Input: part model. Units: mm. Frame: model coordinates. Face numbers are marked on the shaded views. A direction names the side the tool comes from. Give positions to 0.01 mm unless a question says otherwise; leave off trailing zeros. Loops run counter-clockwise (first coordinate to the right, second up) from the corner with the lowest first, then second, coordinate; pieces in that order, holes last.
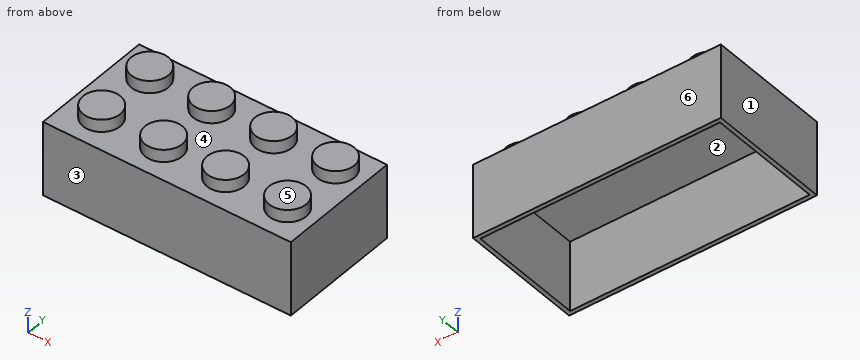
from build123d import *

# Parameters (mm, degrees)
F0_W     = 60
F0_H     = 30
F1_DEPTH = 18
F2_T     = -1
F3_R     = 4.5
F4_DEPTH = 3


with BuildPart() as f1:
    # F0 (on Top) → F1 (new body)
    with BuildSketch(Plane.XY):
        with Locations((30, 15)):
            Rectangle(F0_W, F0_H)
    extrude(amount=F1_DEPTH)

    # F2
    f2_openings = [f1.faces().sort_by_distance(p)[0] for p in [
        (30, 15, 0),
    ]]
    offset(amount=F2_T, openings=f2_openings)

    # F3 (on face) → F4 (join)
    with BuildSketch(Plane.XY.offset(18)):
        with Locations((8, 8)):
            Circle(F3_R)
        with Locations((23, 8)):
            Circle(F3_R)
        with Locations((8, 23)):
            Circle(F3_R)
        with Locations((23, 23)):
            Circle(F3_R)
        with Locations((38, 23)):
            Circle(F3_R)
        with Locations((53, 8)):
            Circle(F3_R)
        with Locations((38, 8)):
            Circle(F3_R)
        with Locations((53, 23)):
            Circle(F3_R)
    extrude(amount=F4_DEPTH)


solid = f1.part
(1) Ray query, probe 1 along Y at (x, z) = (5, 6); probe 2 along X at (y, z) = (18, 12.5); probe 3 along Z at (x, y) = (29, 27.75). Return the intervals inside material, ascending.
Values follow:
probe 1: y = 0 to 1, 29 to 30
probe 2: x = 0 to 1, 59 to 60
probe 3: z = 17 to 18
(2) Reachability of the marked faces 1 and 2 from +Z, -Z, +X, -X, +Y, -Y: full face, straight path, thin tool, end or side. Return the list, or none.
Values follow:
face 1: +Z, -Z, -X, +Y, -Y
face 2: -Z
(3) Cut plane C-C (z = 12). Return the cut outline in (x, y).
Values follow:
outline: (0, 0) - (60, 0) - (60, 30) - (0, 30) - close; hole (1, 1) - (59, 1) - (59, 29) - (1, 29) - close
(4) Cut plane D-D (x = 8). Return the cut outline in (y, z), and give its area (3 significant figures).
Values follow:
outline: (0, 0) - (1, 0) - (1, 17) - (29, 17) - (29, 0) - (30, 0) - (30, 18) - (27.5, 18) - (27.5, 21) - (18.5, 21) - (18.5, 18) - (12.5, 18) - (12.5, 21) - (3.5, 21) - (3.5, 18) - (0, 18) - close
area: 118 mm2
(5) Mould query, pull axis Y, two halves, no side actions, for the marked faces 3, 4, 5 and 6. Classes: +Y half, -Y half, draft (parallel to the pull), parting line (faces both ways), or undercut.
Values follow:
face 3: -Y half
face 4: undercut
face 5: draft
face 6: +Y half
(6) Cut plane A-A (z = 19.75). Return the cut outline in (x, y), and give its area (3 significant figures).
Values follow:
outline: circle Ø9 at (8, 8); circle Ø9 at (8, 23); circle Ø9 at (23, 8); circle Ø9 at (23, 23); circle Ø9 at (38, 8); circle Ø9 at (38, 23); circle Ø9 at (53, 8); circle Ø9 at (53, 23)
area: 509 mm2
(7) Cut plane B-B (y = 8). Return the cut outline in (x, z), and give its area (3 significant figures).
Values follow:
outline: (0, 0) - (1, 0) - (1, 17) - (59, 17) - (59, 0) - (60, 0) - (60, 18) - (57.5, 18) - (57.5, 21) - (48.5, 21) - (48.5, 18) - (42.5, 18) - (42.5, 21) - (33.5, 21) - (33.5, 18) - (27.5, 18) - (27.5, 21) - (18.5, 21) - (18.5, 18) - (12.5, 18) - (12.5, 21) - (3.5, 21) - (3.5, 18) - (0, 18) - close
area: 202 mm2
(8) Pin query (flat end, axial travel): pin 1 Ø14 at (x, y) = (17.5, 14.5) entering from -Z. Return the tip coordinate at first contact, or that it passes through.
Values follow:
pin 1: stops at z = 17
